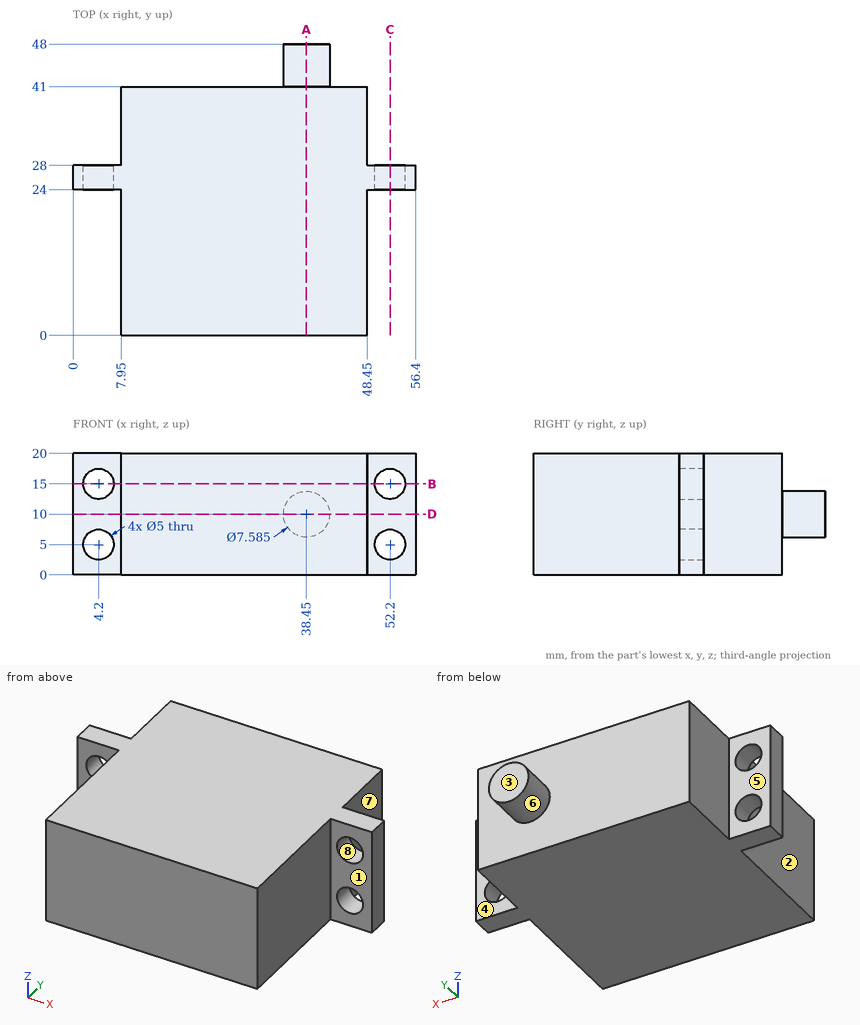
Study the drawing (mm; zero at the part's minimum x, y, z) and answer. A direction names the side the tool comes from. Coordinates: 2 decimals unless noted, no trailing zeros. Write each loop counter-clockwise with the first axis right and the second up, starting at its lowest first coordinate (ties: lowest second). Pieces come first, ordered by that corner, then holes. Notation, with made-up numbers: (63, 2) - (118, 2) arc R12 ccw to (118, 24) - close; hole circle Ø11 at (-23, 14). An arc over 180 degrees is marked (long way). One line per question, with ' | ' between items.
1) Flat-ended cylindrical pins translate along their axes: P1, Ø5, axis at y = 8.5, z = 12.5, coming from the -X side; P2, Ø10, axis at y = 12, z = 12, coming from the +X side; P3, Ø6.5, axis at x = 4.5, z = 14.5, coming from the +Y side; P4, Ø4, axis at x = 38, z = 5.5, coming from the -Y side. Find the tip coordinate at first contact, or state that the pin passes through.
Checks:
P1: x = 7.95 | P2: x = 48.45 | P3: y = 28 | P4: y = 0
2) Find section B-B, the plane z = 15. Determine the outline of the cut face in (x, y), and give its area (3 significant figures).
Checks:
outline: (0, 24) - (1.7, 24) - (1.7, 28) - (0, 28) - close; (6.7, 24) - (7.95, 24) - (7.95, 0) - (48.45, 0) - (48.45, 24) - (49.7, 24) - (49.7, 28) - (48.45, 28) - (48.45, 41) - (7.95, 41) - (7.95, 28) - (6.7, 28) - close; (54.7, 24) - (56.4, 24) - (56.4, 28) - (54.7, 28) - close | area: 1,680 mm2
3) Consider probe 1 along Z at (x, y) = (4, 27); probe 2 along X at (y, z) = (25.6, 5); probe 3 along Y at (x, z) = (14.5, 10.75). Determine where each line is inside the solid, lowest interval first. Write a range as [from, to].
Checks:
probe 1: [0, 2.51], [7.49, 12.51], [17.49, 20] | probe 2: [0, 1.7], [6.7, 49.7], [54.7, 56.4] | probe 3: [0, 41]
4) Find section A-A, the plane x = 38.45. Determine the outline of the cut face in (y, z), and give its area (3 significant figures).
Checks:
outline: (0, 0) - (41, 0) - (41, 6.21) - (48, 6.21) - (48, 13.79) - (41, 13.79) - (41, 20) - (0, 20) - close | area: 873 mm2
5) Find section D-D, the plane z = 10. Determine the outline of the cut face in (x, y).
Checks:
outline: (0, 24) - (7.95, 24) - (7.95, 0) - (48.45, 0) - (48.45, 24) - (56.4, 24) - (56.4, 28) - (48.45, 28) - (48.45, 41) - (42.24, 41) - (42.24, 48) - (34.66, 48) - (34.66, 41) - (7.95, 41) - (7.95, 28) - (0, 28) - close
6) Find section C-C, the plane x = 52.2. Determine the outline of the cut face in (y, z), and give its area (3 significant figures).
Checks:
outline: (24, 0) - (28, 0) - (28, 2.5) - (24, 2.5) - close; (24, 7.5) - (28, 7.5) - (28, 12.5) - (24, 12.5) - close; (24, 17.5) - (28, 17.5) - (28, 20) - (24, 20) - close | area: 40.0 mm2
7) For the marked faces 1, 2, 3, 4 and 5, determine the directions among +Z, -Z, +X, -X, +Y, -Y from which every point of the face is accessible in a straight line to the end or side of a thin tool.
Checks:
face 1: +Z, -Z, +X, -Y | face 2: +Z, -Z, -X, -Y | face 3: +Z, -Z, +X, -X, +Y | face 4: +Z, -Z, +X, +Y | face 5: +Z, -Z, -X, +Y
8) The mould has two halves that part along X. Classify the marked faces 6, 7 and 8: +X half, -X half, draft (parallel to the pull), parting line (faces both ways), or undercut.
Checks:
face 6: parting line | face 7: +X half | face 8: undercut
